Input: dimensioned drawing with shaded views. Units: mm. Origin: part minimum x, y, z. Round coordinates to 2 decimals unless told otherwise and drop trailing zeros. Write each loop counter-clockwise with the first axis right and the second up, starting at its lowest first coordinate (ties: lowest second). Pieces come first, ordered by that corner, then holes. Notation, with made-up numbers: M 15.25,18.25 L 71.25,18.25 A34 ccw 71.25,49.25 Z; hole C -2.75,25 d8. An arc over 180 degrees is marked long. Answer in a Markdown table with one row per item. Add a question column.
Item 1: Material intervals for probe 1 along X at (y, z) = (40, 4); probe 2 along Y at (x, z) = (65, 6.75); probe 3 along X at (y, z) = (9, 2), sorted ascending.
Item 2: Cut plane C-C on z = 5. Return loops of the section in (x, y), and give its area (3 significant figures).
Item 3: Cut plane B-B on y = 40. Return loops of the section in (x, z).
Item 4: Contact query for a flat-ended pin moving along its axis: pin 1 (10 mm diameter, centred on x = 38, y = 11.5, fed in from -Z). Output: stop coordinate, or through.
Item 5: Cut plane A-A on x = 15. Return loops of the section in (y, z), and give its area (3 significant figures).
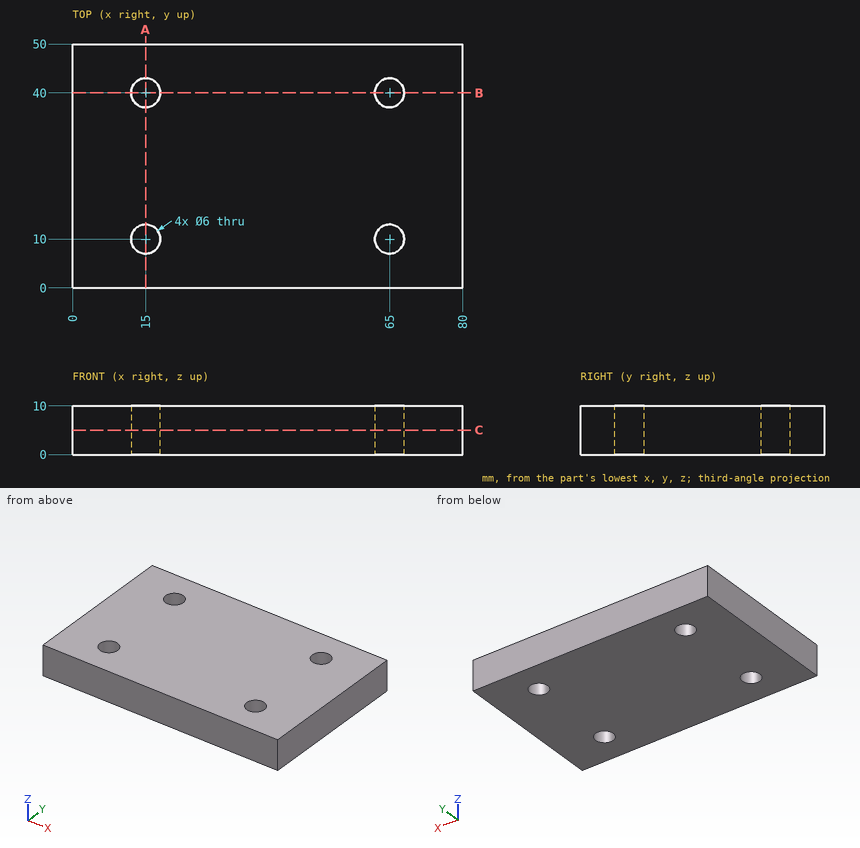
Results below:
| question | item | result |
|---|---|---|
| 1 | probe 1 | 0 to 12, 18 to 62, 68 to 80 |
| 1 | probe 2 | 0 to 7, 13 to 37, 43 to 50 |
| 1 | probe 3 | 0 to 12.17, 17.83 to 62.17, 67.83 to 80 |
| 2 | outline | M 0,0 L 80,0 L 80,50 L 0,50 Z; hole C 15,10 d6; hole C 15,40 d6; hole C 65,10 d6; hole C 65,40 d6 |
| 2 | area | 3,890 mm2 |
| 3 | outline | M 0,0 L 12,0 L 12,10 L 0,10 Z; M 18,0 L 62,0 L 62,10 L 18,10 Z; M 68,0 L 80,0 L 80,10 L 68,10 Z |
| 4 | pin 1 | z = 0 |
| 5 | outline | M 0,0 L 7,0 L 7,10 L 0,10 Z; M 13,0 L 37,0 L 37,10 L 13,10 Z; M 43,0 L 50,0 L 50,10 L 43,10 Z |
| 5 | area | 380 mm2 |
